```python
from build123d import *

# Parameters (mm, degrees)
SKETCH_R  = 4.5
PAD_DEPTH = 1.5
FILLET_R  = 2


with BuildPart() as part:
    # Sketch → Pad (new body, symmetric)
    with BuildSketch(Plane.XZ):
        Polygon((-42.5, 110), (42.5, 110), (42.5, 74), (18, 74), (18, 0), (-18, 0), (-18, 74), (-42.5, 74), align=None)
        with Locations((-27.5, 92)):
            Circle(SKETCH_R, mode=Mode.SUBTRACT)
        with Locations((27.5, 92)):
            Circle(SKETCH_R, mode=Mode.SUBTRACT)
        with Locations((0, 20)):
            Circle(SKETCH_R, mode=Mode.SUBTRACT)
        with Locations((0, 50)):
            Circle(SKETCH_R, mode=Mode.SUBTRACT)
    extrude(amount=PAD_DEPTH, both=True)

    # Fillet
    fillet_edges = [part.edges().sort_by_distance(p)[0] for p in [
        (42.5, 0, 110),
        (42.5, 0, 74),
        (18, 0, 74),
        (-18, 0, 74),
        (-42.5, 0, 74),
        (-42.5, 0, 110),
        (18, 0, 0),
        (-18, 0, 0),
    ]]
    fillet(fillet_edges, radius=FILLET_R)


solid = part.part
```
The listing builds one solid part. Answer for the finished solid, in the listing's coordinates (mm). A direction names the side the tool comes from. Coordinates: 2 decimals unless noted, no trailing zeros. Write each loop counter-clockwise with the first axis right and the second up, starting at its lowest first coordinate (ties: lowest second). Pieces come first, ordered by that corner, then holes. Notation, with made-up numbers: (46, -33) - (68, -33) arc R22 ccw to (68, 6) - close; hole circle Ø4 at (66, 56). An arc over 180 degrees is marked (long way). One line per item, written item: value.
1) For a pull along Z with two mould halves and no side action, classify faces 4 (the flat face through (30, 0, 74)), 5 (the flat face through (-1, 0, 110)), 6 (the cylindrical face through (2.419, 0.021, 23.794)), 7 (the flat face through (-18, 0, 37)) as pulls with the +Z half, pulls with the -Z half, needs draft (parallel to the pull), parting line crosses it, or undercut.
Geometry check:
face 4: pulls with the -Z half
face 5: pulls with the +Z half
face 6: undercut
face 7: needs draft
2) Find section A-A (x = 0). Give the vertices of the cut face in (y, z).
Geometry check:
outline: (-1.5, 0) - (1.5, 0) - (1.5, 15.5) - (-1.5, 15.5) - close; (-1.5, 24.5) - (1.5, 24.5) - (1.5, 45.5) - (-1.5, 45.5) - close; (-1.5, 54.5) - (1.5, 54.5) - (1.5, 110) - (-1.5, 110) - close
3) Each of these flat-tipped pins is pushed along its axis until it touches: pin 1 Ø1.5 at (y, z) = (0, 25.5) entering from +X; pin 2 Ø0.9 at (x, y) = (30, -0.5) entering from -Z; pin 3 Ø14.5 at (x, z) = (0, 50) entering from +Y. Where does it stop, or does it pass through?
Geometry check:
pin 1: stops at x = 18
pin 2: stops at z = 74
pin 3: stops at y = 1.5
4) Consider line 1 along Z through (x, y) = (0, -0.2); line 2 along Z through (x, y) = (-27, -1.1); line 3 along X through (y, z) = (-0.2, 50.5). Determine where each line is inside the solid, lowest interval first. Write a range as from..to.
Geometry check:
line 1: z = 0..15.5, 24.5..45.5, 54.5..110
line 2: z = 74..87.53, 96.47..110
line 3: x = -18..-4.47, 4.47..18
5) Find section C-C (y = 1). Give the vertices of the cut face in (x, z), and give its area (3 significant figures).
Geometry check:
outline: (-42.5, 76) arc R2 ccw to (-40.5, 74) - (-20, 74) arc R2 cw to (-18, 72) - (-18, 2) arc R2 ccw to (-16, 0) - (16, 0) arc R2 ccw to (18, 2) - (18, 72) arc R2 cw to (20, 74) - (40.5, 74) arc R2 ccw to (42.5, 76) - (42.5, 108) arc R2 ccw to (40.5, 110) - (-40.5, 110) arc R2 ccw to (-42.5, 108) - close; hole circle Ø9 at (-27.5, 92); hole circle Ø9 at (0, 20); hole circle Ø9 at (0, 50); hole circle Ø9 at (27.5, 92)
area: 5,470 mm2
6) Find section D-D (z = 50). Give the vertices of the cut face in (x, y).
Geometry check:
outline: (-18, -1.5) - (-4.5, -1.5) - (-4.5, 1.5) - (-18, 1.5) - close; (4.5, -1.5) - (18, -1.5) - (18, 1.5) - (4.5, 1.5) - close
7) A tool of negligible diameter and unlimited length cuts with its end or side. For faces 1 (the flat face through (42.5, 0, 92)), 2 (the flat face through (18, 0, 37)), 3 (the flat face through (-30, 0, 74)), from which of +Z, -Z, +X, -X, +Y, -Y can it reach the whole face along a straight path? Write none if from no direction.
Geometry check:
face 1: +Z, -Z, +X, +Y, -Y
face 2: -Z, +X, +Y, -Y
face 3: -Z, -X, +Y, -Y
8) Find section B-B (z = 92). Give the vertices of the cut face in (x, y).
Geometry check:
outline: (-42.5, -1.5) - (-32, -1.5) - (-32, 1.5) - (-42.5, 1.5) - close; (-23, -1.5) - (23, -1.5) - (23, 1.5) - (-23, 1.5) - close; (32, -1.5) - (42.5, -1.5) - (42.5, 1.5) - (32, 1.5) - close
